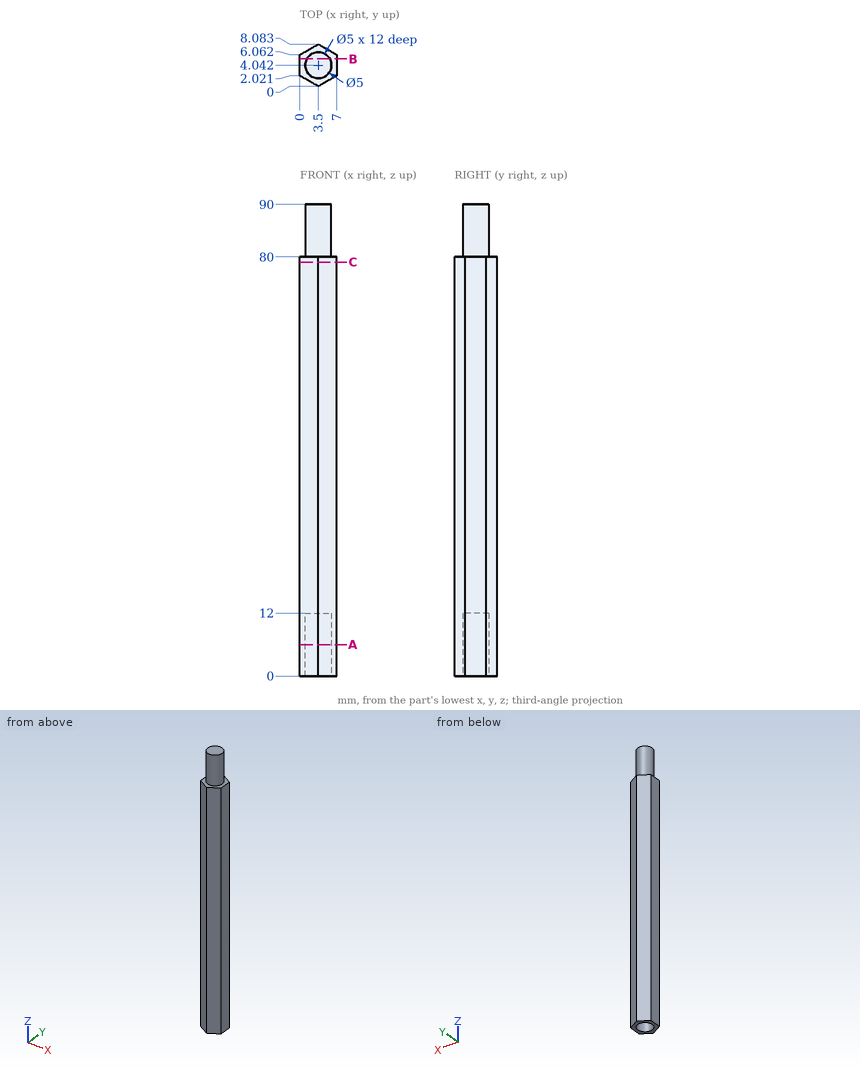
Print and shaded views of the part. All mm, measured from the part's lowest x, y and z. Coordinates: 2 decimals unless noted, no trailing zeros. Order: outer loops, then holes, each group sorted by start corner. A loop starts at its lowest first (then second) coordinate and runs counter-clockwise, first axis right, second up.
Item 1: Saw through at A-A on z = 6. List the corners of the cut face in (x, y), then the cut area to 3 significant figures.
Filled in:
outline: (0, 2.02) - (3.5, 0) - (7, 2.02) - (7, 6.06) - (3.5, 8.08) - (0, 6.06) - close; hole circle Ø5 at (3.5, 4.04)
area: 22.8 mm2
Item 2: Drop flat-ended pins along their axis: pin 1 Ø1 at (x, z) = (1.5, 55.5) entering from +Y; pin 2 Ø3 at (x, z) = (4.5, 60) entering from +Y; pin 3 Ø3 at (x, z) = (6, 72) entering from +Y (1 decimal). Give the stop position or say it passes through.
Filled in:
pin 1: stops at y = 7.22
pin 2: stops at y = 8.08
pin 3: stops at y = 7.5
Item 3: Saw through at C-C on z = 79. List the corners of the cut face in (x, y).
Filled in:
outline: (0, 2.02) - (3.5, 0) - (7, 2.02) - (7, 6.06) - (3.5, 8.08) - (0, 6.06) - close
Item 4: Saw through at B-B on y = 5.25. List the corners of the cut face in (x, z).
Filled in:
outline: (0, 0) - (1.31, 0) - (1.31, 12) - (5.69, 12) - (5.69, 0) - (7, 0) - (7, 80) - (5.69, 80) - (5.69, 90) - (1.31, 90) - (1.31, 80) - (0, 80) - close
Item 5: Drill centre lines: L1, parallel to Z at x = 2.75, y = 2; L2, parallel to Z at x = 2.75, y = 7.25; L3, parallel to X at y = 7.25, z = 72.5 (1 decimal). Where is each one in solid material? Low to high.
Filled in:
L1: z = 12 to 90
L2: z = 0 to 80
L3: x = 2.1 to 4.9
